For this review, take the finished solid that the model builds, in its own axes (mm). A direction names the side the tool comes from. Round coordinates to 2 decimals unless told otherwise and drop trailing zeros. Use one line per item in the form item = value. Start each with the question number.
Item 1: For line 1 (Z direction, x = 1.25, y = -2.15); line 2 (Z direction, x = -0.5, y = -0.1) (3 decimals); line 3 (Z direction, x = -6.25, y = 0.95), list the stretches that pass through material, from the lowest coordinate up. Write a range as [from, to].
Item 2: For P1, Ø3, axis at y = 0.5, z = 5.5, coming from the -X side; P2, Ø3, axis at y = -1.5, z = 3.5, coming from the -X side; P3, Ø1.7, axis at y = 0.5, z = 4.5, coming from the +X side; P4, Ø2, axis at x = -8.5, z = -2, coming from the -Y side, all flat-tipped, find the tip position at first contact; note any pin that passes through.
Item 3: For faces 4 (the flat face through (-4.47, 1.63, -7.91)), 5 (the flat face through (-4.53, 1.63, 7.91)), 6 (the flat face through (-2.5, -2, -4)), 7 (the flat face through (-2.05, 0, -6)), 8 (the flat face through (0, 0.04, -7.05)), list the 3-axis set-ups (+Z, -Z, +X, -X, +Y, -Y) from which the entire face can be reached by the end or side of a thin tool; tool diameter is ignored.
Item 4: Draft analysis for pull direction X (two halves, no side actions). For faces 1 (the flat face through (-2.5, -2, 4)), 2 (the flat face through (0, 0, -3.5)), 3 (the flat face through (-2.5, -2, -8)), state which applies: released by +X, released by -X, zero draft, split by the parting line, or undercut.
from build123d import *

# Parameters (mm, degrees)
SKETCH005_W             = 5
SKETCH005_H             = 5
PAD_DEPTH               = 2.5
POCKET_DEPTH            = 2.501
POCKET_DEPTH_BACK       = 2.501
BODY002_PLACEMENT_ANGLE = 180


with BuildPart() as part:
    # AdditivePipe001: sweep along a path in Sketch002
    with BuildLine(Plane.XZ) as additivepipe001_path:
        Line((0, -6), (6.500025, -6))
        ThreePointArc((6.500025, -6), (10.742649, -4.242632), (12.5, 0))
        ThreePointArc((12.5, 0), (10.742641, 4.242641), (6.5, 6))
        Line((6.5, 6), (-2.5e-05, 6))
    # Sketch003 → AdditivePipe001 (sweep)
    with BuildSketch(Plane.YZ):
        with BuildLine():
            ThreePointArc((2.5, -6), (0, -3.5), (-2.5, -6))
            Line((-2.5, -6), (-2.5, -7.301418))
            Line((-2.5, -7.301418), (-0.788247, -8.5))
            Line((-0.788247, -8.5), (0.788247, -8.5))
            Line((0.788247, -8.5), (2.5, -7.301418))
            Line((2.5, -7.301418), (2.5, -6))
        make_face()
    sweep(path=additivepipe001_path.line)

    # Sketch005 → Pad (new body, symmetric)
    with BuildSketch(Plane.YZ):
        with Locations((0, 6)):
            Rectangle(SKETCH005_W, SKETCH005_H)
        with Locations((0, -6)):
            Rectangle(SKETCH005_W, SKETCH005_H)
    extrude(amount=PAD_DEPTH, both=True)

    # Sketch004 → Pocket (cut, two sides)
    with BuildSketch(Plane.XZ) as pocket_sk:
        with BuildLine():
            Line((-1.790135, 6.960364), (1.840135, 7.139636))
            ThreePointArc((2.05, 6.93988), (1.98789, 7.084747), (1.840135, 7.139636))
            Line((2.05, 6.93988), (2.05, 5.06012))
            ThreePointArc((1.840135, 4.860364), (1.98789, 4.915253), (2.05, 5.06012))
            Line((1.840135, 4.860364), (-1.790135, 5.039636))
            ThreePointArc((-1.790135, 5.039636), (-1.93789, 4.984747), (-2, 4.83988))
            Line((-2, 3), (-2, 4.83988))
            Line((-2.5, 3), (-2, 3))
            Line((-2.5, 9), (-2.5, 3))
            Line((-2, 9), (-2.5, 9))
            Line((-2, 7.16012), (-2, 9))
            ThreePointArc((-2, 7.16012), (-1.93789, 7.015253), (-1.790135, 6.960364))
        make_face()
        with BuildLine():
            Line((1.790012, -5.239501), (-1.790013, -5.060499))
            ThreePointArc((-1.790013, -5.060499), (-1.937845, -5.11534), (-2, -5.26025))
            Line((-2, -5.26025), (-2, -6.73975))
            ThreePointArc((-2, -6.73975), (-1.937845, -6.88466), (-1.790012, -6.939501))
            Line((-1.790012, -6.939501), (1.790012, -6.760499))
            ThreePointArc((2, -6.96025), (1.937845, -6.81534), (1.790012, -6.760499))
            Line((2, -6.96025), (2, -9))
            Line((2, -9), (-3, -9))
            Line((-3, -9), (-3, -3))
            Line((-3, -3), (2, -3))
            Line((2, -3), (2, -5.03975))
            ThreePointArc((1.790012, -5.239501), (1.937845, -5.18466), (2, -5.03975))
        make_face()
    extrude(amount=-POCKET_DEPTH, mode=Mode.SUBTRACT)
    extrude(pocket_sk.sketch, amount=POCKET_DEPTH_BACK, mode=Mode.SUBTRACT)


with BuildPart() as part_1:
    # Body002 placement: moved
    add(part.part.rotate(Axis((0, 0, 0), (0, 1, 0)), BODY002_PLACEMENT_ANGLE))


solid = part_1.part
Calculated:
q1.line_1 = [-8.5, -6.99], [-5.01, -3.5], [5.09, 6.91]
q1.line_2 = [-8.5, -7.073], [-4.927, -3.5], [5.175, 6.825]
q1.line_3 = [-8.39, -3.69], [3.69, 8.39]
q2.P1 = -14
q2.P2 = -14.72
q2.P3 = 2
q2.P4 = -1.24
q3.face_4 = -Z, -X, +Y
q3.face_5 = +Z, -X, +Y
q3.face_6 = -Y
q3.face_7 = +X, +Y, -Y
q3.face_8 = +Y, -Y
q4.face_1 = undercut
q4.face_2 = zero draft
q4.face_3 = released by -X
